Here's how the part is built. I have some questions about the finished solid (model axes, mm). A direction names the side the tool comes from. Give positions to 0.01 mm unless a question says otherwise; leave off trailing zeros. Write each loop counter-clockwise with the first axis right and the second up, starting at its lowest first coordinate (ties: lowest second). Pieces come first, ordered by that corner, then holes. Notation, with made-up numbers: (-11.75, 80) - (4.25, 80) arc R9 ccw to (4.25, 92) - close; hole circle Ø10 at (66, 62.25). An arc over 180 degrees is marked (long way). Write each question's results on one line, items separated by ' | '. Start each with the question number.
Item 1: Suppose I cut it at A-A on z = 7.5. List the corners of the cut face in (x, y) for me, then the cut area to 3 significant figures.
Item 2: Which directions (+Z, -Z, +X, -X, +Y, -Y) give clear straight access to the entire face, cutting with the end or side of a thin tool? Please do faces 5 (the flat face through (10, 7, 0)), 6 (the flat face through (1.5, 12, 8)).
Item 3: We'd pull the mould along X, two halves only. Please class faces 1 (the flat face through (10, 15, 7)), 2 (the cylindrical face through (16.156, 7.605, 7.337)), 3 (the flat face through (0, 7, 8)), 4 (the flat face through (20, 7, 8)): +X half, -X half, draft (parallel to the pull), parting line (faces both ways), or undercut.
Item 4: Please list where these lines run through material, in increasing order: line 1 along X through (y, z) = (8.5, 7.5); line 2 along X through (y, z) = (7, 7.5); line 3 along Z through (x, y) = (17, 13).
```python
from build123d import *

# Parameters (mm, degrees)
CROQUIS1_W              = 20
CROQUIS1_H              = 15
SALIENTE_EXTRUIR1_DEPTH = 15
CROQUIS2_R              = 0.75
CORTAR_EXTRUIR1_DEPTH   = 16
CROQUIS2_3_W            = 0.5
CROQUIS2_3_H            = 2
CORTAR_EXTRUIR2_DEPTH   = 7


with BuildPart() as part:
    # Croquis1 → Saliente-Extruir1 (new body)
    with BuildSketch(Plane(origin=(0, 0, 0), x_dir=(1, 0, 0), z_dir=(0, 1, 0))):
        with Locations((10, -7.5)):
            Rectangle(CROQUIS1_W, CROQUIS1_H)
    extrude(amount=SALIENTE_EXTRUIR1_DEPTH)

    # Croquis2 → Cortar-Extruir1 (cut, through all)
    with BuildSketch(Plane(origin=(0, 15, 0), x_dir=(1, 0, 0), z_dir=(0, 1, 0))):
        with Locations(Location((16.888623538, -7.5, 0), (0, 0, 270))):  # turned: the seam where the file's is
            Circle(CROQUIS2_R)
    extrude(amount=-CORTAR_EXTRUIR1_DEPTH, mode=Mode.SUBTRACT)

    # Croquis2_3 → Cortar-Extruir2 (cut)
    with BuildSketch(Plane(origin=(0, 15, 0), x_dir=(1, 0, 0), z_dir=(0, 1, 0))):
        with Locations((1.25, -7.5)):
            Rectangle(CROQUIS2_3_W, CROQUIS2_3_H)
    extrude(amount=-CORTAR_EXTRUIR2_DEPTH, mode=Mode.SUBTRACT)


solid = part.part
```
Checked values:
1) outline: (0, 0) - (16.14, 0) - (16.14, 15) - (1.5, 15) - (1.5, 8) - (1, 8) - (1, 15) - (0, 15) - close; (17.64, 0) - (20, 0) - (20, 15) - (17.64, 15) - close | area: 274 mm^2
2) face 5: -Z, +X, -X, +Y, -Y | face 6: +Y
3) face 1: draft | face 2: undercut | face 3: -X half | face 4: +X half
4) line 1: x = 0 to 1, 1.5 to 16.14, 17.64 to 20 | line 2: x = 0 to 16.14, 17.64 to 20 | line 3: z = 0 to 6.76, 8.24 to 15
